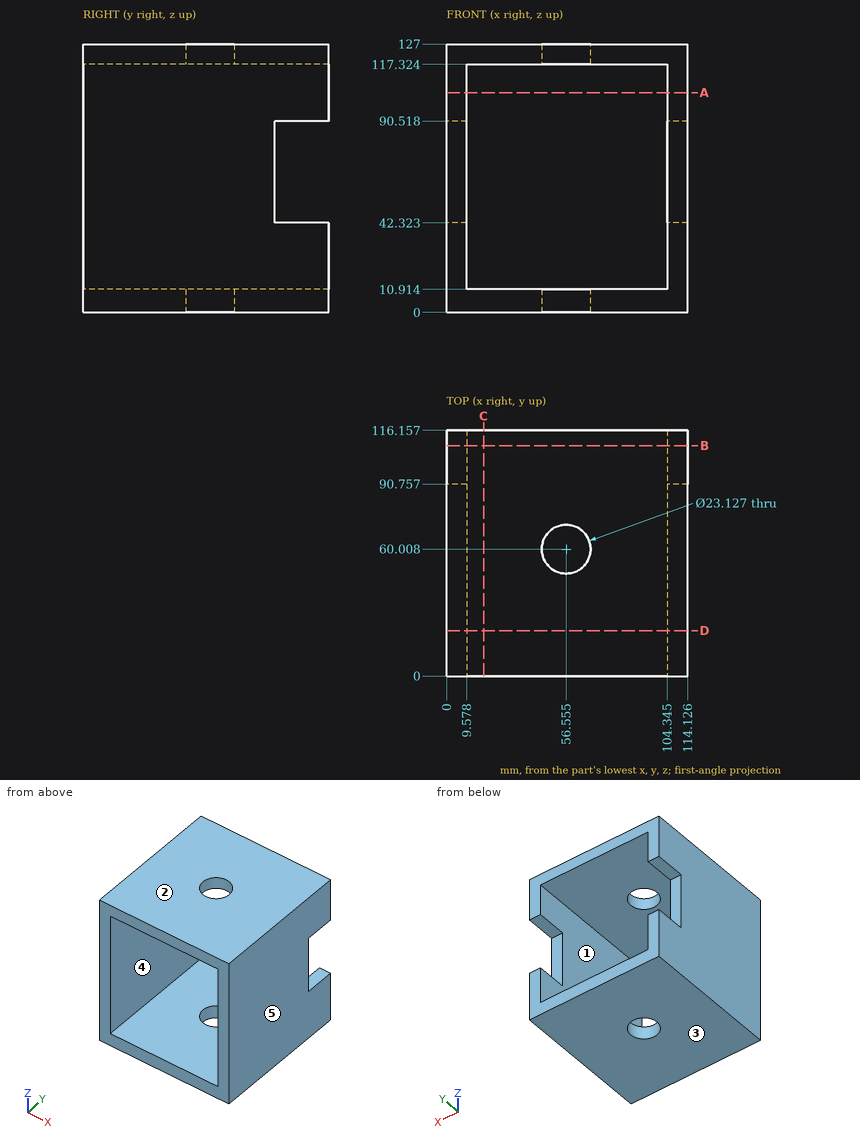
Can you work these out from the drawing? Everything is in mm from the part's minimum corner. A direction names the side the tool comes from. Give positions to 0.01 mm unless a question says otherwise; leave off trailing zeros. Loops run counter-clockwise (first coordinate to the right, second up) from the corner with the lowest first, then second, coordinate; pieces in that order, holes last. Notation, with made-up numbers: (16, -33.5) -> (47, -33.5) arc R9 ccw to (47, -23.5) -> close; hole circle Ø2 at (79.5, 10). An arc over 180 degrees is marked (long way). Return JSON: item names as keys, results as strings.
Q1. I need wall thicknesses on probe 1 along X at (y, z) = (68, 61) (1 decimal); probe 2 along Z at (x, y) = (75, 47) (1 decimal); probe 3 along Y at (x, z) = (49.5, 10.5) (1 decimal). Which ranges of each line are inside material? Lowest first, please.
Checks:
{"probe 1": "x = 0 to 9.6, 104.3 to 114.1", "probe 2": "z = 0 to 10.9, 117.3 to 127", "probe 3": "y = 0 to 50.8, 69.2 to 116.2"}
Q2. I want a section at D-D, the plane y = 21.5. List the corners of the cut face in (x, z) for me (1 decimal).
Checks:
{"outline": "(0, 0) -> (114.1, 0) -> (114.1, 127) -> (0, 127) -> close; hole (9.6, 10.9) -> (104.3, 10.9) -> (104.3, 117.3) -> (9.6, 117.3) -> close"}
Q3. I want a section at A-A, the plane z = 104. List the corners of the cut face in (x, y) for me (1 decimal).
Checks:
{"outline": "(0, 0) -> (9.6, 0) -> (9.6, 116.2) -> (0, 116.2) -> close; (104.3, 0) -> (114.1, 0) -> (114.1, 116.2) -> (104.3, 116.2) -> close"}
Q4. I want a section at C-C, the plane x = 17.5. List the corners of the cut face in (y, z) for me (1 decimal), then the cut area to 3 significant figures.
Checks:
{"outline": "(0, 0) -> (116.2, 0) -> (116.2, 10.9) -> (0, 10.9) -> close; (0, 117.3) -> (116.2, 117.3) -> (116.2, 127) -> (0, 127) -> close", "area": "2,390 mm2"}
Q5. For pin 1 Ø11 at (x, z) = (109, 65.5) entering from +Y, with a flat end and sliding along its axis, tell me the tip position at first contact or that it passes through.
Checks:
{"pin 1": "stops at y = 90.76"}
Q6. We'd pull the mould along X, two halves only. Please class the marked faces 3, 4 and 5: released by +X, released by -X, zero draft, split by the parting line, or undercut.
Checks:
{"face 3": "zero draft", "face 4": "undercut", "face 5": "released by +X"}
Q7. I want a section at B-B, the plane y = 109. List the corners of the cut face in (x, z) for me (1 decimal).
Checks:
{"outline": "(0, 0) -> (114.1, 0) -> (114.1, 42.3) -> (104.3, 42.3) -> (104.3, 10.9) -> (9.6, 10.9) -> (9.6, 42.3) -> (0, 42.3) -> close; (0, 90.5) -> (9.6, 90.5) -> (9.6, 117.3) -> (104.3, 117.3) -> (104.3, 90.5) -> (114.1, 90.5) -> (114.1, 127) -> (0, 127) -> close"}
Q8. On a 3-axis mill with a long thin cutter (end or side, diameter ignored), from which of +Z, -Z, +X, -X, +Y, -Y can I reach the whole of each face in a straight line? I mean the marked faces 1 and 2. Say none if no direction works.
Checks:
{"face 1": "+Y, -Y", "face 2": "+Z, +X, -X, +Y, -Y"}
